The listing builds one solid part. Answer for the finished solid, in the listing's coordinates (mm). Face numbers are marked on the shaded views. A direction names the side the tool comes from. Give positions to 0.01 mm unless a question says otherwise; leave off trailing zeros. Loops run counter-clockwise (first coordinate to the right, second up) from the corner with the lowest first, then second, coordinate; pieces in that order, holes last. Notation, with made-up numbers: M -29,-31 L 4,-31 A22 cw 4,-3 Z; hole C 44,8.5 d6. An arc over 180 degrees is marked long. One line per item, written item: value. Start each with the question number.
Q1. A cutting plane is placed at B-B, the plane x = -85.5. Determine the outline of the cut face in (y, z), and give its area (3 significant figures).
Q2. A cutting plane is placed at D-D, the plane x = 62. Determine the outline of the cut face in (y, z).
Q3. A cutting plane is placed at A-A, the plane z = 271. Determine the outline of the cut face in (x, y), and give its area (3 significant figures).
Q4. Consider L1, parallel to X at y = 35, z = 225; L2, parallel to X at y = 41.5, z = 225. Determine where each line is inside the solid, lowest interval first.
Q5. A cutting plane is placed at C-C, the plane z = 39.5. Determine the outline of the cut face in (x, y).
Q6. For the marked faces 1, 2 and 3, determine the directions among +Z, -Z, +X, -X, +Y, -Y from which every point of the face is accessible in a straight line to the end or side of a thin tool.
Q7. Flat-ended cylindrical pins translate along their axes: pin 1 (8 mm diameter, centred on x = 93, z = 144, fed in from -Y); pin 2 (1.5 mm diameter, centred on x = -39, z = 246.5, fed in from +Y); pin 3 (1.5 mm diameter, centred on x = -6, z = 295.5, fed in from +Y). Find the tip coordinate at first contact, or state that the pin passes through.
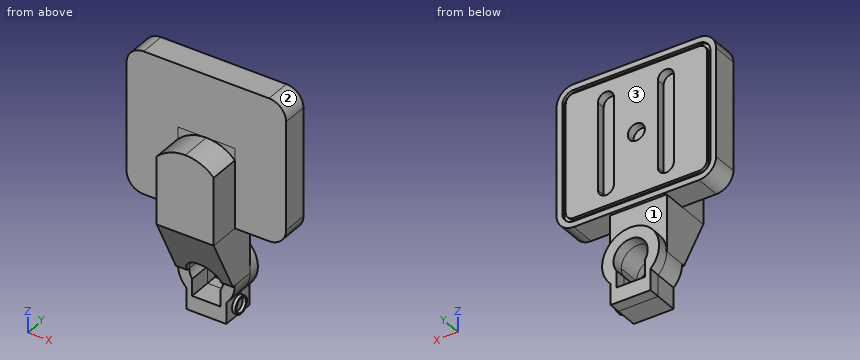
from build123d import *
from build123d.topology import SkipClean

# Parameters (mm, degrees)
BOSS_EXTRUDE1_DEPTH      = 40
CUT_EXTRUDE1_DEPTH       = 66
BOSS_EXTRUDE2_START      = -55
BOSS_EXTRUDE2_DEPTH      = 95
CUT_EXTRUDE2_DEPTH       = 256
BOSS_EXTRUDE3_DEPTH      = 5
BOSS_EXTRUDE3_DEPTH_BACK = 40
BOSS_EXTRUDE4_DEPTH      = 20
CUT_EXTRUDE3_DEPTH       = 5
BOSS_EXTRUDE5_DEPTH      = 5
SKETCH9_R                = 15
CUT_EXTRUDE5_DEPTH       = 15
SKETCH10_W               = 100
SKETCH10_H               = 55
BOSS_EXTRUDE6_DEPTH      = 140
CUT_EXTRUDE6_DEPTH       = 55
SKETCH12_R               = 15
BOSS_EXTRUDE7_DEPTH      = 6
SKETCH13_R               = 12.5
CUT_EXTRUDE7_DEPTH       = 6


with BuildPart() as part:
    # Sketch1 → Boss-Extrude1 (new body)
    with BuildSketch(Plane(origin=(0, 0, 0), x_dir=(1, 0, 0), z_dir=(0, 1, 0))):
        with BuildLine():
            Line((-35, 73), (35, 73))
            Line((35, 73), (35, 35.707142143))
            ThreePointArc((35, 35.707142143), (0, -50), (-35, 35.707142143))
            Line((-35, 35.707142143), (-35, 73))
        make_face()
    extrude(amount=BOSS_EXTRUDE1_DEPTH)

    # Sketch2 → Cut-Extrude1 (cut)
    with BuildSketch(Plane(origin=(0, 40, 0), x_dir=(1, 0, 0), z_dir=(0, 1, 0))):
        with BuildLine():
            Line((-25.015, 16.587646005), (-25.015, 46.245))
            Line((-25.015, 46.245), (25.015, 46.245))
            Line((25.015, 46.245), (25.015, 16.587646005))
            ThreePointArc((25.015, 16.587646005), (0, -30.015), (-25.015, 16.587646005))
        make_face()
    extrude(amount=-CUT_EXTRUDE1_DEPTH, mode=Mode.SUBTRACT)

    # Sketch3 → Boss-Extrude2 (add)
    with SkipClean():  # the faces are left unmerged after this step: merging them gives an invalid solid
        with BuildSketch(Plane(origin=(0, 0, 0), x_dir=(1, 0, 0), z_dir=(0, 1, 0)).offset(BOSS_EXTRUDE2_START)):
            with BuildLine():
                Line((30.015, 0), (50, 0))
                Line((50, 0), (50, -100))
                Line((50, -100), (-50, -100))
                Line((-50, -100), (-50, 0))
                Line((-50, 0), (-30.015, 0))
                ThreePointArc((-30.015, 0), (0, -30.015), (30.015, 0))
            make_face()
        extrude(amount=BOSS_EXTRUDE2_DEPTH)

    # Sketch4 → Cut-Extrude2 (cut)
    with SkipClean():  # the faces are left unmerged after this step: merging them gives an invalid solid
        with BuildSketch(Plane(origin=(50, 0, 0), x_dir=(0, 0, -1), z_dir=(1, 0, 0))):
            Polygon((-100, -55), (0, -5.02758566), (0, -55), align=None)
        extrude(amount=-CUT_EXTRUDE2_DEPTH, mode=Mode.SUBTRACT)

    # Sketch5 → Boss-Extrude3 (add, two sides: drawn at the far end of the back side and taken through both)
    with SkipClean():  # the faces are left unmerged after this step: merging them gives an invalid solid
        with BuildSketch(Plane(origin=(0, 40, 0), x_dir=(1, 0, 0), z_dir=(0, 1, 0)).offset(-BOSS_EXTRUDE3_DEPTH_BACK)):
            with BuildLine():
                Line((-110, -350), (110, -350))
                ThreePointArc((110, -350), (131.213203436, -341.213203436), (140, -320))
                Line((140, -320), (140, -130))
                ThreePointArc((140, -130), (131.213203436, -108.786796564), (110, -100))
                Line((110, -100), (-110, -100))
                ThreePointArc((-110, -100), (-131.213203436, -108.786796564), (-140, -130))
                Line((-140, -130), (-140, -320))
                ThreePointArc((-140, -320), (-131.213203436, -341.213203436), (-110, -350))
            make_face()
        extrude(amount=BOSS_EXTRUDE3_DEPTH + BOSS_EXTRUDE3_DEPTH_BACK)

    # Sketch6 → Boss-Extrude4 (add)
    with SkipClean():  # the faces are left unmerged after this step: merging them gives an invalid solid
        with BuildSketch(Plane(origin=(0, 40, 0), x_dir=(1, 0, 0), z_dir=(0, 1, 0))):
            with BuildLine():
                Line((-35, 35.707142143), (-35, 73))
                Line((-35, 73), (35, 73))
                Line((35, 73), (35, 35.707142143))
                ThreePointArc((35, 35.707142143), (0, -50), (-35, 35.707142143))
            make_face()
            with BuildLine():
                Line((-25.015, 16.587646005), (-25.015, 46.245))
                Line((-25.015, 46.245), (25.015, 46.245))
                Line((25.015, 46.245), (25.015, 16.587646005))
                ThreePointArc((25.015, 16.587646005), (0, -30.015), (-25.015, 16.587646005))
            make_face(mode=Mode.SUBTRACT)
        extrude(amount=BOSS_EXTRUDE4_DEPTH)

    # Sketch7 → Cut-Extrude3 (cut)
    with SkipClean():  # the faces are left unmerged after this step: merging them gives an invalid solid
        with BuildSketch(Plane(origin=(0, 45, 0), x_dir=(1, 0, 0), z_dir=(0, 1, 0))):
            with BuildLine():
                Line((130, -320), (130, -130))
                ThreePointArc((130, -130), (124.142135624, -115.857864376), (110, -110))
                Line((110, -110), (-110, -110))
                ThreePointArc((-110, -110), (-124.142135624, -115.857864376), (-130, -130))
                Line((-130, -130), (-130, -320))
                ThreePointArc((-130, -320), (-124.142135624, -334.142135624), (-110, -340))
                Line((-110, -340), (110, -340))
                ThreePointArc((110, -340), (124.142135624, -334.142135624), (130, -320))
            make_face()
        extrude(amount=-CUT_EXTRUDE3_DEPTH, mode=Mode.SUBTRACT)

    # Sketch8 → Boss-Extrude5 (add)
    with SkipClean():  # the faces are left unmerged after this step: merging them gives an invalid solid
        with BuildSketch(Plane(origin=(0, 40, 0), x_dir=(1, 0, 0), z_dir=(0, 1, 0))):
            with BuildLine():
                Line((124, -320), (124, -130))
                ThreePointArc((124, -130), (119.899494937, -120.100505063), (110, -116))
                Line((110, -116), (-110, -116))
                ThreePointArc((-110, -116), (-119.899494937, -120.100505063), (-124, -130))
                Line((-124, -130), (-124, -320))
                ThreePointArc((-124, -320), (-119.899494937, -329.899494937), (-110, -334))
                Line((-110, -334), (110, -334))
                ThreePointArc((110, -334), (119.899494937, -329.899494937), (124, -320))
            make_face()
        extrude(amount=BOSS_EXTRUDE5_DEPTH)

    # Sketch9 → Cut-Extrude5 (cut)
    with SkipClean():  # the faces are left unmerged after this step: merging them gives an invalid solid
        with BuildSketch(Plane(origin=(0, 45, 0), x_dir=(1, 0, 0), z_dir=(0, 1, 0))):
            with Locations(Location((0, -225, 0), (0, 0, 270))):
                Circle(SKETCH9_R)
            with BuildLine():
                Line((-65.823520443, -301.518564523), (-65.823520443, -148.481435477))
                ThreePointArc((-65.823520443, -148.481435477), (-51.823520443, -134.481435477), (-37.823520443, -148.481435477))
                Line((-37.823520443, -148.481435477), (-37.823520443, -301.518564523))
                ThreePointArc((-37.823520443, -301.518564523), (-51.823520443, -315.518564523), (-65.823520443, -301.518564523))
            make_face()
            with BuildLine():
                Line((39.386204855, -301.518564523), (39.386204855, -148.481435477))
                ThreePointArc((39.386204855, -148.481435477), (53.386204855, -134.481435477), (67.386204855, -148.481435477))
                Line((67.386204855, -148.481435477), (67.386204855, -301.518564523))
                ThreePointArc((67.386204855, -301.518564523), (53.386204855, -315.518564523), (39.386204855, -301.518564523))
            make_face()
        extrude(amount=-CUT_EXTRUDE5_DEPTH, mode=Mode.SUBTRACT)

    # Sketch10 → Boss-Extrude6 (add)
    with SkipClean():  # the faces are left unmerged after this step: merging them gives an invalid solid
        with BuildSketch(Plane.XY.offset(100)):
            with Locations((0, -27.5)):
                Rectangle(SKETCH10_W, SKETCH10_H)
        extrude(amount=BOSS_EXTRUDE6_DEPTH)

    # Sketch11 → Cut-Extrude6 (cut)
    with SkipClean():  # the faces are left unmerged after this step: merging them gives an invalid solid
        with BuildSketch(Plane.XZ.offset(55)):
            with BuildLine():
                Line((50, 240), (0, 240))
                ThreePointArc((0, 240), (27.117470016, 234.534043883), (50, 218.989794856))
                Line((50, 218.989794856), (50, 240))
            make_face()
            with BuildLine():
                Line((0, 240), (-50, 240))
                Line((-50, 240), (-50, 218.989794856))
                ThreePointArc((-50, 218.989794856), (-27.117470016, 234.534043883), (0, 240))
            make_face()
        extrude(amount=-CUT_EXTRUDE6_DEPTH, mode=Mode.SUBTRACT)

    # Sketch12 → Boss-Extrude7 (add)
    with SkipClean():  # the faces are left unmerged after this step: merging them gives an invalid solid
        with BuildSketch(Plane(origin=(35, 0, 0), x_dir=(0, 0, -1), z_dir=(1, 0, 0))):
            with Locations(Location((54.353571071, 30, 0), (0, 0, 180))):
                Circle(SKETCH12_R)
        extrude(amount=BOSS_EXTRUDE7_DEPTH)

    # Sketch13 → Cut-Extrude7 (cut)
    with SkipClean():  # the faces are left unmerged after this step: merging them gives an invalid solid
        with BuildSketch(Plane(origin=(41, 0, 0), x_dir=(0, 0, -1), z_dir=(1, 0, 0))):
            with Locations((54.353571071, 30)):
                Circle(SKETCH13_R)
        extrude(amount=-CUT_EXTRUDE7_DEPTH, mode=Mode.SUBTRACT)


solid = part.part
Answer block:
1. outline: M 0,100 L 45,100 L 45,110 L 40,110 L 40,116 L 45,116 L 45,334 L 40,334 L 40,340 L 45,340 L 45,350 L 0,350 Z
1. area: 11,200 mm^2
2. outline: M 0,100 L 45,100 L 45,110 L 40,110 L 40,116 L 45,116 L 45,137.45 L 30,137.45 L 30,312.55 L 45,312.55 L 45,334 L 40,334 L 40,340 L 45,340 L 45,350 L 0,350 Z
3. outline: M -140,0 L 140,0 L 140,45 L 130,45 L 130,40 L 124,40 L 124,45 L 67.39,45 L 67.39,30 L 39.39,30 L 39.39,45 L -37.82,45 L -37.82,30 L -65.82,30 L -65.82,45 L -124,45 L -124,40 L -130,40 L -130,45 L -140,45 Z
3. area: 11,700 mm^2
4. L1: -140 to -65.82, -37.82 to -15, 15 to 39.39, 67.39 to 140
4. L2: -140 to -130, -124 to -65.82, -37.82 to -15, 15 to 39.39, 67.39 to 124, 130 to 140
5. outline: M -50,-24.77 L 50,-24.77 L 50,40 L 30.66,40 L 30.66,60 L -30.66,60 L -30.66,40 L -50,40 Z
6. face 1: +Y
6. face 2: +Z, +X, +Y, -Y
6. face 3: +Z, +X, -X, +Y
7. pin 1: y = 0
7. pin 2: y = 30
7. pin 3: y = 45
